Source: CAD feature listing. Evaluate the final solid. Frame: model axes, mm. Coordinates: 2 decimals unless noted, no trailing zeros. Order: outer loops, then holes, each group sorted by start corner. A loop starts at its lowest first (then second) coordinate and runs counter-clockwise, first axis right, second up.
```python
from build123d import *

# Parameters (mm, degrees)
SKETCH_1_W          = 265
SKETCH_1_H          = 121.5
EXTRUDE_1_DEPTH     = 3
SKETCH_2_R          = 10
CUT_EXTRUDE_1_DEPTH = 10
SKETCH_3_W          = 70.6
SKETCH_3_H          = 49.6
CUT_EXTRUDE_2_DEPTH = 3
FILLET_1_R          = 2
SKETCH_4_R          = 1.498589197
CUT_EXTRUDE_3_DEPTH = 10
SKETCH_5_R          = 1.5
CUT_EXTRUDE_4_DEPTH = 42
SKETCH_6_W          = 40.5
SKETCH_6_H          = 27
CUT_EXTRUDE_5_DEPTH = 22
FILLET_2_R          = 2


with BuildPart() as part:
    # 草图1 → 凸台-拉伸1 (new body)
    with BuildSketch(Plane.XY):
        Rectangle(SKETCH_1_W, SKETCH_1_H)
    extrude(amount=EXTRUDE_1_DEPTH)

    # 草图2 → 切除-拉伸1 (cut)
    with BuildSketch(Plane(origin=(0, 0, 0), x_dir=(-1, 0, 0), z_dir=(0, 0, -1))):
        with Locations((55, 35.75)):
            Circle(SKETCH_2_R)
    cut_extrude_1 = extrude(amount=-CUT_EXTRUDE_1_DEPTH, mode=Mode.SUBTRACT)

    # 镜向1: 切除-拉伸1 across plane
    add(cut_extrude_1.mirror(Plane(origin=(0, 0, 0), x_dir=(0, 0, 1), z_dir=(1, 0, 0))), mode=Mode.SUBTRACT)

    # 草图3 → 切除-拉伸2 (cut)
    with BuildSketch(Plane.XY.offset(3)):
        with Locations((-65.5, -21.75)):
            Rectangle(SKETCH_3_W, SKETCH_3_H)
    extrude(amount=-CUT_EXTRUDE_2_DEPTH, mode=Mode.SUBTRACT)

    # 圆角1
    fillet_1_edges = [part.edges().sort_by_distance(p)[0] for p in [
        (-100.8, 3.05, 1.5),
        (-100.8, -46.55, 1.5),
        (-30.2, -46.55, 1.5),
        (-30.2, 3.05, 1.5),
    ]]
    fillet(fillet_1_edges, radius=FILLET_1_R)

    # 草图4 → 切除-拉伸3 (cut)
    with BuildSketch(Plane.XY.offset(3)):
        with Locations((-29, -49.75)):
            Circle(SKETCH_4_R)
        with Locations((-29, 6.25)):
            Circle(SKETCH_4_R)
        with Locations((-102, -49.75)):
            Circle(SKETCH_4_R)
        with Locations((-102, 6.25)):
            Circle(SKETCH_4_R)
    extrude(amount=-CUT_EXTRUDE_3_DEPTH, mode=Mode.SUBTRACT)

    # 草图5 → 切除-拉伸4 (cut)
    with BuildSketch(Plane.XY.offset(3)):
        with Locations((95, 16.25)):
            Circle(SKETCH_5_R)
        with Locations((95, -51.75)):
            Circle(SKETCH_5_R)
        with Locations((0, -51.75)):
            Circle(SKETCH_5_R)
        with Locations((0, 16.25)):
            Circle(SKETCH_5_R)
    extrude(amount=-CUT_EXTRUDE_4_DEPTH, mode=Mode.SUBTRACT)

    # 草图6 → 切除-拉伸5 (cut)
    with BuildSketch(Plane.XY.offset(3)):
        with Locations((25.25, -33.25)):
            Rectangle(SKETCH_6_W, SKETCH_6_H)
        with Locations((25.25, -2.25)):
            Rectangle(SKETCH_6_W, SKETCH_6_H)
        with Locations((69.75, -2.25)):
            Rectangle(SKETCH_6_W, SKETCH_6_H)
        with Locations((69.75, -33.25)):
            Rectangle(SKETCH_6_W, SKETCH_6_H)
    extrude(amount=-CUT_EXTRUDE_5_DEPTH, mode=Mode.SUBTRACT)

    # 圆角2
    fillet_2_edges = [part.edges().sort_by_distance(p)[0] for p in [
        (49.5, -19.75, 1.5),
        (90, -19.75, 1.5),
        (90, -46.75, 1.5),
        (49.5, -46.75, 1.5),
        (49.5, 11.25, 1.5),
        (90, 11.25, 1.5),
        (90, -15.75, 1.5),
        (49.5, -15.75, 1.5),
        (5, -15.75, 1.5),
        (5, 11.25, 1.5),
        (45.5, 11.25, 1.5),
        (45.5, -15.75, 1.5),
        (45.5, -19.75, 1.5),
        (45.5, -46.75, 1.5),
        (5, -46.75, 1.5),
        (5, -19.75, 1.5),
    ]]
    fillet(fillet_2_edges, radius=FILLET_2_R)


solid = part.part
```
Q1. Pin query (flat end, axial travel): P1, Ø1.8, axis at x = -102, y = -49.75, coming from the +Z side. Return the tip coordinate at first contact, or that it passes through.
Solutions:
P1: passes through
Q2. Section query A-A on x = 55. Output: boundary loops of the cut face in (y, z).
Solutions:
outline: (-60.75, 0) - (-46.75, 0) - (-46.75, 3) - (-60.75, 3) - close; (-19.75, 0) - (-15.75, 0) - (-15.75, 3) - (-19.75, 3) - close; (11.25, 0) - (25.75, 0) - (25.75, 3) - (11.25, 3) - close; (45.75, 0) - (60.75, 0) - (60.75, 3) - (45.75, 3) - close
Q3. Section query D-D on y = -28.5. Output: boundary loops of the cut face in (x, z).
Solutions:
outline: (-132.5, 0) - (-100.8, 0) - (-100.8, 3) - (-132.5, 3) - close; (-30.2, 0) - (5, 0) - (5, 3) - (-30.2, 3) - close; (45.5, 0) - (49.5, 0) - (49.5, 3) - (45.5, 3) - close; (90, 0) - (132.5, 0) - (132.5, 3) - (90, 3) - close
Q4. Material intervals for line 1 along Y through (x, z) = (-102, 2.1); line 2 along Y through (x, z) = (87, 0.8); line 3 along X through (y, z) = (16, 2.6), sorted ascending.
Solutions:
line 1: y = -60.75 to -51.25, -48.25 to 4.75, 7.75 to 60.75
line 2: y = -60.75 to -46.75, -19.75 to -15.75, 11.25 to 60.75
line 3: x = -132.5 to -1.48, 1.48 to 93.52, 96.48 to 132.5
Q5. Section query B-B on y = 35.75. Output: boundary loops of the cut face in (x, z).
Solutions:
outline: (-132.5, 0) - (-65, 0) - (-65, 3) - (-132.5, 3) - close; (-45, 0) - (45, 0) - (45, 3) - (-45, 3) - close; (65, 0) - (132.5, 0) - (132.5, 3) - (65, 3) - close
Q6. Section query C-C on x = -35. Output: boundary loops of the cut face in (y, z).
Solutions:
outline: (-60.75, 0) - (-46.55, 0) - (-46.55, 3) - (-60.75, 3) - close; (3.05, 0) - (60.75, 0) - (60.75, 3) - (3.05, 3) - close
Q7. Pull-direction query (Y, two-part tool) for faces 1 (the cylindrical face through (47.06, 29.67, 1.48)), 2 (the flat face through (-2, 1, 3)); classes: pulls with the +Y half, pulls with the -Y half, needs draft (parallel to the pull), parting line crosses it, or undercut.
Solutions:
face 1: undercut
face 2: needs draft
